```python
from build123d import *

# Parameters (mm, degrees)
F1_DEPTH = 3
F2_R     = 5
F3_DEPTH = 3


with BuildPart() as f1:
    # F0 (on Top) → F1 (new body)
    with BuildSketch(Plane.XY):
        Polygon((-69, 98.640618), (-249, 98.640618), (-249, -132.831599), (0, -132.831599), (0, 22.168401), align=None)
    extrude(amount=F1_DEPTH)

    # F2 (on face) → F3 (cut)
    with BuildSketch(Plane.XY.offset(3)):
        with Locations((-35, -72.831599)):
            Circle(F2_R)
    extrude(amount=-F3_DEPTH, mode=Mode.SUBTRACT)


solid = f1.part
```
Check sheet for the modelled part. Datum: model origin and axes. Units: mm. Round coordinates to 2 decimals unless told otherwise and drop trailing zeros. Loops run counter-clockwise (first coordinate to the right, second up) from the corner with the lowest first, then second, coordinate; pieces in that order, holes last. Notation, with made-up numbers: (-39.5, 84) - (17.5, 84) arc R17 cw to (17.5, 98) - close; hole circle Ø10 at (-24, 49.25). An arc over 180 degrees is marked (long way). Write item = value, one per line. Start each with the question number.
Q1. Thickness scan on L1, parallel to Y at x = -35, z = 0.95; L2, parallel to X at y = 53, z = 2.2; L3, parallel to Y at x = -61, z = 2. Record the ranges inside material, lowest first.
Q2. Section check C-C (y = 50). Record the boundary of the cut face in (x, z).
Q3. Section check B-B (z = 1). Record the boundary of the cut face in (x, y), plus the area to 3 significant figures.
Q4. Section check A-A (x = -35). Record the boundary of the cut face in (y, z), plus the area to 3 significant figures.
Q5. Release check for a two-part mould opening along X. For faces 1 (the face through (-34.02, 59.87, 1.48)), 2 (the face through (-126, -15, 3)), 3 (the face through (-36.084, -77.713, 1.521)) record: pulls with the +X half, pulls with the -X half, needs draft (parallel to the pull), parting line crosses it, or undercut.
Derived:
q1.L1 = -132.83 to -77.83, -67.83 to 60.96
q1.L2 = -249 to -27.82
q1.L3 = -132.83 to 89.77
q2.outline = (-249, 0) - (-25.11, 0) - (-25.11, 3) - (-249, 3) - close
q3.outline = (-249, -132.83) - (0, -132.83) - (0, 22.17) - (-69, 98.64) - (-249, 98.64) - close; hole circle Ø10 at (-35, -72.83)
q3.area = 54,900 mm^2
q4.outline = (-132.83, 0) - (-77.83, 0) - (-77.83, 3) - (-132.83, 3) - close; (-67.83, 0) - (60.96, 0) - (60.96, 3) - (-67.83, 3) - close
q4.area = 551 mm^2
q5.face_1 = pulls with the +X half
q5.face_2 = needs draft
q5.face_3 = undercut
